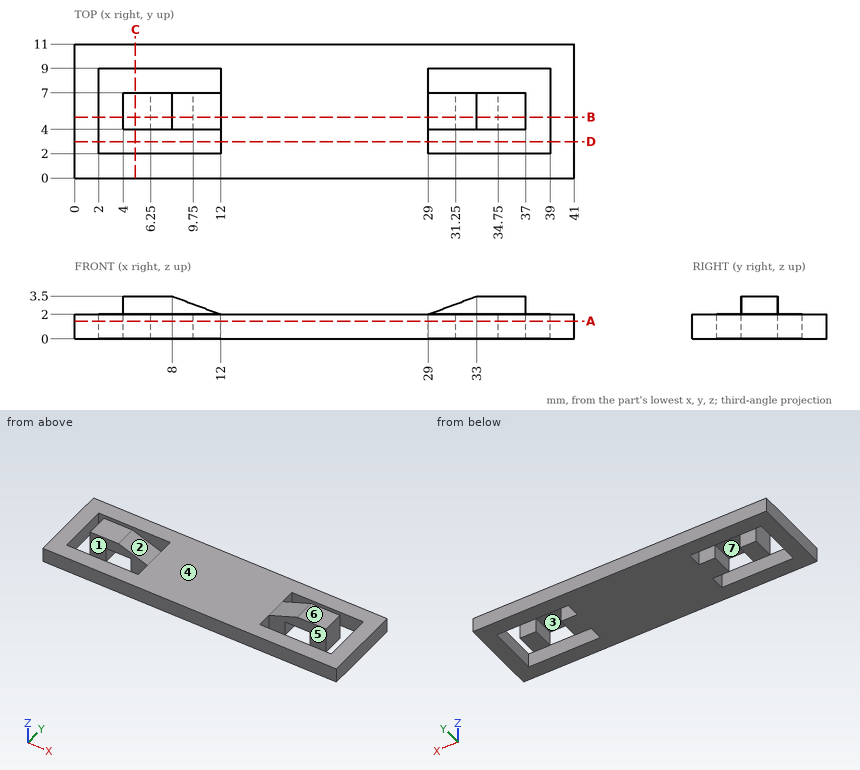
For this review, use the dimensioned drawing (mm, ordinates from the lowest corner) and the shaded views. A direction names the side the tool comes from. Round coordinates to 2 decimals unless told otherwise and drop trailing zeros. Order: outer loops, then holes, each group sorted by start corner. A loop starts at its lowest first (then second) coordinate and runs counter-clockwise, first axis right, second up. Notation, with made-up numbers: M 5,41 L 47,41 A14 ccw 47,52 Z; hole C 12,66 d10. An arc over 180 degrees is marked long. Use a Markdown table: item, result. Add a question column.
Item 1: Add section B-B, the plane y = 5. Give the boundary of the cut face in (x, z), then the cut area to 3 significant figures.
Item 2: Tool access review of the marked faces 1, 2, 3 and 4: name each direction out of +Z, -Z, +X, -X, +Y, -Y from which nothing blocks a thin tool from reaching the whole face with its end or side.
Item 3: Add section C-C, the plane x = 5. Give the boundary of the cut face in (y, z), then the cut area to 3 significant figures.
Item 4: Insertion check: pin 1 (2 mm diameter, centred on y = 6.5, z = 0.5, fed in from -X); pin 2 (4 mm diameter, centred on x = 16, y = 6.5, fed in from +Z). Each pin has a flat end and moves straight along its axis. Give the tip position at first contact, or say it passes through.
Item 5: Add section A-A, the plane z = 1.45. Give the boundary of the cut face in (x, y).
Item 6: To check wall thickness, follow line 1 along X through (y, z) = (2.5, 1.75); line 2 along Y through (x, z) = (36.5, 0.55); line 3 along X through (y, z) = (5, 1.4). State the ranges of each line that lie inside material, in increasing order.
Item 7: Mouldability with a two-part tool opening along X and no side actions: class the marked faces 5, 6 and 7 as released by +X, released by -X, zero draft, split by the parting line, or undercut.
Item 8: Add section D-D, the plane y = 3. Give the boundary of the cut face in (x, z), then the cut area to 3 significant figures.
Geometry results:
| question | item | result |
|---|---|---|
| 1 | outline | M 0,0 L 2,0 L 2,2 L 0,2 Z; M 4,0 L 6.25,0 L 6.25,2 L 9.75,2 L 9.75,0 L 31.25,0 L 31.25,2 L 34.75,2 L 34.75,0 L 37,0 L 37,3.5 L 33,3.5 L 29,2 L 12,2 L 8,3.5 L 4,3.5 Z; M 39,0 L 41,0 L 41,2 L 39,2 Z |
| 1 | area | 78.0 mm² |
| 2 | face 1 | +Z, -Z |
| 2 | face 2 | +Z, +Y, -Y |
| 2 | face 3 | -Z |
| 2 | face 4 | +Z |
| 3 | outline | M 0,0 L 2,0 L 2,2 L 0,2 Z; M 4,0 L 7,0 L 7,3.5 L 4,3.5 Z; M 9,0 L 11,0 L 11,2 L 9,2 Z |
| 3 | area | 18.5 mm² |
| 4 | pin 1 | stops at x = 0 |
| 4 | pin 2 | stops at z = 2 |
| 5 | outline | M 0,0 L 41,0 L 41,11 L 0,11 Z; M 4,4 L 6.25,4 L 6.25,7 L 4,7 Z; M 34.75,4 L 37,4 L 37,7 L 34.75,7 Z; hole M 2,2 L 12,2 L 12,4 L 9.75,4 L 9.75,7 L 12,7 L 12,9 L 2,9 Z; hole M 29,2 L 39,2 L 39,9 L 29,9 L 29,7 L 31.25,7 L 31.25,4 L 29,4 Z |
| 6 | line 1 | x = 0 to 2, 12 to 29, 39 to 41 |
| 6 | line 2 | y = 0 to 2, 4 to 7, 9 to 11 |
| 6 | line 3 | x = 0 to 2, 4 to 6.25, 9.75 to 31.25, 34.75 to 37, 39 to 41 |
| 7 | face 5 | undercut |
| 7 | face 6 | zero draft |
| 7 | face 7 | undercut |
| 8 | outline | M 0,0 L 2,0 L 2,2 L 0,2 Z; M 12,0 L 29,0 L 29,2 L 12,2 Z; M 39,0 L 41,0 L 41,2 L 39,2 Z |
| 8 | area | 42.0 mm² |
